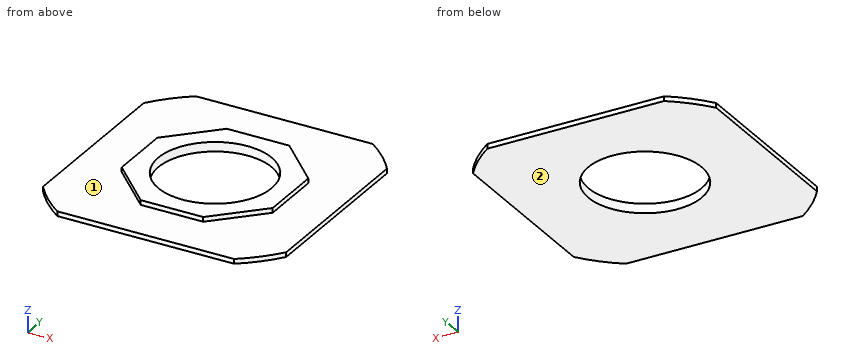
from build123d import *

# Parameters (mm, degrees)
SKETCH1_R           = 38.5
SKETCH1_W           = 203.947710216
SKETCH1_H           = 203.947710216
BOSS_EXTRUDE1_DEPTH = 3.175
SKETCH1_3_R         = 38.5
BOSS_EXTRUDE2_DEPTH = 6.35
SKETCH6_W           = 203.947710216
SKETCH6_H           = 203.947710216
CUT_EXTRUDE1_DEPTH  = 15


with BuildPart() as part:
    # Sketch1 → Boss-Extrude1 (new body)
    with BuildSketch(Plane.XY):
        Polygon((51.2, -21.207734394), (51.2, 21.207734394), (21.207734394, 51.2), (-21.207734394, 51.2), (-51.2, 21.207734394), (-51.2, -21.207734394), (-21.207734394, -51.2), (21.207734394, -51.2), align=None)
        Circle(SKETCH1_R, mode=Mode.SUBTRACT)
        Rectangle(SKETCH1_W, SKETCH1_H)
        Polygon((51.2, 21.207734394), (21.207734394, 51.2), (-21.207734394, 51.2), (-51.2, 21.207734394), (-51.2, -21.207734394), (-21.207734394, -51.2), (21.207734394, -51.2), (51.2, -21.207734394), align=None, mode=Mode.SUBTRACT)
    extrude(amount=BOSS_EXTRUDE1_DEPTH)

    # Sketch1_3 → Boss-Extrude2 (add)
    with BuildSketch(Plane.XY):
        Polygon((51.2, -21.207734394), (51.2, 21.207734394), (21.207734394, 51.2), (-21.207734394, 51.2), (-51.2, 21.207734394), (-51.2, -21.207734394), (-21.207734394, -51.2), (21.207734394, -51.2), align=None)
        Circle(SKETCH1_3_R, mode=Mode.SUBTRACT)
    extrude(amount=BOSS_EXTRUDE2_DEPTH)

    # Sketch6 → Cut-Extrude1 (cut)
    with BuildSketch(Plane(origin=(0, 0, 0), x_dir=(-1, 0, 0), z_dir=(0, 0, -1))):
        Rectangle(SKETCH6_W, SKETCH6_H)
        with BuildLine():
            ThreePointArc((-59.981247069, 82.5), (-72.124891681, 72.124891681), (-82.5, 59.981247069))
            Line((-82.5, 59.981247069), (-82.5, -59.981247069))
            ThreePointArc((-82.5, -59.981247069), (-72.124891681, -72.124891681), (-59.981247069, -82.5))
            Line((-59.981247069, -82.5), (59.981247069, -82.5))
            ThreePointArc((59.981247069, -82.5), (72.124891681, -72.124891681), (82.5, -59.981247069))
            Line((82.5, -59.981247069), (82.5, 59.981247069))
            ThreePointArc((82.5, 59.981247069), (72.124891681, 72.124891681), (59.981247069, 82.5))
            Line((59.981247069, 82.5), (-59.981247069, 82.5))
        make_face(mode=Mode.SUBTRACT)
    extrude(amount=-CUT_EXTRUDE1_DEPTH, mode=Mode.SUBTRACT)


solid = part.part
CAD build for the part. Positions are in the model's coordinates, mm. Face numbers are marked on the shaded views. A direction names the side the tool comes from. Give positions to 0.01 mm unless a question says otherwise; leave off trailing zeros. Loops run counter-clockwise (first coordinate to the right, second up) from the corner with the lowest first, then second, coordinate; pieces in that order, holes last. Notation, with made-up numbers: M 44,46.25 L 80,46.25 A30 cw 80,72.25 Z; hole C -17.75,2 d11. An arc over 180 degrees is marked long. One line per question, with ' | ' between items. Start each with the question number.
1. 3-axis set-ups, long thin cutter, end or side, ignore diameter. For the marked faces 1 and 2: which of +Z, -Z, +X, -X, +Y, -Y reach the whole face in a straight line?
2. Saw through at A-A on z = 2. Give the cut face in (x, y).
3. Saw through at D-D on x = 57. Give the cut face in (y, z) (3 decimals), plus the area to 3 significant figures.
4. Probe L1, parallel to Y at x = 0, z = 4.75; L2, parallel to Z at x = -60, y = -46.5 (3 decimals); L3, parallel to X at y = -20, z = 3. List the from-to ranges inside material, lowest first. Write a range as from..to.
5. Saw through at B-B on x = 0. Give the cut face in (y, z) (3 decimals), plus the area to 3 significant figures.
6. Flat gauge pins, fed straight in: pin 1 (1 mm diameter, centred on x = 7, z = 5, fed in from -Y); pin 2 (2.5 mm diameter, centred on y = 2.5, z = 5, fed in from +X); pin 3 (1 mm diameter, centred on x = 5, z = 5, fed in from +Y). Where does each tip first touch, or does it go through?
Result sheet:
1) face 1: +Z | face 2: -Z, +X, -X, +Y, -Y
2) outline: M -82.5,-59.98 A102 ccw -59.98,-82.5 L 59.98,-82.5 A102 ccw 82.5,-59.98 L 82.5,59.98 A102 ccw 59.98,82.5 L -59.98,82.5 A102 ccw -82.5,59.98 Z; hole C 0,0 d77
3) outline: M -82.5,0 L 82.5,0 L 82.5,3.175 L -82.5,3.175 Z | area: 524 mm^2
4) L1: y = -51.2..-38.5, 38.5..51.2 | L2: z = 0..3.175 | L3: x = -82.5..-32.9, 32.9..82.5
5) outline: M -82.5,0 L -38.5,0 L -38.5,6.35 L -51.2,6.35 L -51.2,3.175 L -82.5,3.175 Z; M 38.5,0 L 82.5,0 L 82.5,3.175 L 51.2,3.175 L 51.2,6.35 L 38.5,6.35 Z | area: 360 mm^2
6) pin 1: stops at y = -51.2 | pin 2: stops at x = 51.2 | pin 3: stops at y = 51.2
